```python
from build123d import *

# Parameters (mm, degrees)
SKETCH1_R                 = 5.5
BOSS_EXTRUDE1_DEPTH       = 6.35
F_6_CLEARANCE_HOLE1_D     = 3.7973
F_6_CLEARANCE_HOLE1_DEPTH = 6.35


with BuildPart() as part:
    # Sketch1 → Boss-Extrude1 (new body)
    with BuildSketch(Plane(origin=(0, 0, 0), x_dir=(0, 0, -1), z_dir=(1, 0, 0))):
        with BuildLine():
            Line((-19.05, 266.7), (19.05, 266.7))
            ThreePointArc((19.05, 266.7), (87.703033087, 128.539281009), (39.110598571, -17.88612161))
            ThreePointArc((39.110598571, -17.88612161), (37.900092771, -18.755241175), (36.426387255, -18.976341069))
            ThreePointArc((36.426387255, -18.976341069), (23.718766847, -12.493303526), (19.076049666, 0.995898429))
            ThreePointArc((19.076049666, 0.995898429), (19.289830149, 1.986417864), (19.804803607, 2.859133845))
            ThreePointArc((19.804803607, 2.859133845), (58.113146317, 140.316763388), (-19.05, 260.35))
            Line((-19.05, 260.35), (-19.05, 266.7))
        make_face()
        with Locations((38.1, 0)):
            Circle(SKETCH1_R, mode=Mode.SUBTRACT)
    extrude(amount=BOSS_EXTRUDE1_DEPTH)

    # #6 Clearance Hole1
    with Locations(Plane(origin=(6.35, 0, 0), x_dir=(0, 0, -1), z_dir=(1, 0, 0))):
        with Locations((-15.875, 263.525), (0, 263.525), (15.875, 263.525)):
            Hole(F_6_CLEARANCE_HOLE1_D / 2, depth=F_6_CLEARANCE_HOLE1_DEPTH)


solid = part.part
```
Geometry check sheet. Reference: the model listing, model coordinates, mm. Round coordinates to 2 decimals unless told otherwise and drop trailing zeros. Loops run counter-clockwise (first coordinate to the right, second up) from the corner with the lowest first, then second, coordinate; pieces in that order, holes last. Notation, with made-up numbers: (56.5, 69) - (74.5, 69) arc R32 cw to (74.5, 95) - close; hole circle Ø7 at (9, 37). An arc over 180 degrees is marked (long way). Use a Markdown table: item, result.
Q1. Cross-section at C-C on y = 194.5. Record the cut outline in (x, z).
Solutions:
| item | result |
|---|---|
| outline | (0, -71.65) - (6.35, -71.65) - (6.35, -40.53) - (0, -40.53) - close |
Q2. Material ranges on line 1 (Y direction, x = 1.5, z = -39); line 2 (Y direction, x = 4.25, z = -35); line 3 (Y direction, x = 4.5, z = 15), recorded low to high.
Solutions:
| item | result |
|---|---|
| line 1 | y = -18.01 to -5.43, 5.43 to 31.22, 197.38 to 246.61 |
| line 2 | y = -18.8 to -4.54, 4.54 to 24.23, 204.37 to 251.11 |
| line 3 | y = 257.63 to 261.84, 265.21 to 266.7 |
Q3. Draft check along Z on faces 1 (the cylindrical face through (3.131, -12.647, -23.854)), 2 (the flat face through (6.35, 125, -63)), 3 (the cylindrical face through (3.131, 130.749, -87.535)), 4 (the cylindrical face through (3.131, 0.242, -32.605)). Enter one of: released by +Z, released by -Z, zero draft, split by the parting line, or undercut.
Solutions:
| item | result |
|---|---|
| face 1 | released by +Z |
| face 2 | zero draft |
| face 3 | released by -Z |
| face 4 | undercut |
Q4. Cross-section at A-A on z = -24. Record the cut outline in (x, y), plus the area to 3 significant figures.
Solutions:
| item | result |
|---|---|
| outline | (0, -12.81) - (6.35, -12.81) - (6.35, 8.11) - (0, 8.11) - close; (0, 220.49) - (6.35, 220.49) - (6.35, 262.22) - (0, 262.22) - close |
| area | 398 mm2 |
Q5. Cross-section at D-D on z = -75. Record the cut outline in (x, y).
Solutions:
| item | result |
|---|---|
| outline | (0, 42.37) - (6.35, 42.37) - (6.35, 186.23) - (0, 186.23) - close |
Q6. Cross-section at B-B on x = 2. Record the cut outline in (y, z) (3 decimals), plus the area to 3 significant figures.
Solutions:
| item | result |
|---|---|
| outline | (-18.976, -36.426) arc R3.175 ccw to (-17.886, -39.111) arc R202.504 ccw to (266.7, -19.05) - (266.7, 19.05) - (260.35, 19.05) arc R174.365 cw to (2.859, -19.805) arc R3.175 ccw to (0.996, -19.076) arc R19.05 ccw to start; hole circle Ø11 at (0, -38.1); hole circle Ø3.797 at (263.525, -15.875); hole circle Ø3.797 at (263.525, 0); hole circle Ø3.797 at (263.525, 15.875) |
| area | 8,730 mm2 |
Q7. Go/stop test with flat-tipped pins: P1, Ø2, axis at x = 4.5, z = -14, coming from the -Y side; P2, Ø2.5, axis at y = 263.525, z = -15.875, coming from the +X side; P3, Ø2, axis at x = 3.5, y = 206, coming from the -Z side; P4, Ø2, axis at x = 4, z = 0.5, coming from the -Y side. Record where each tip stops, or that it passes through.
Solutions:
| item | result |
|---|---|
| P1 | stops at y = 231.28 |
| P2 | passes through |
| P3 | stops at z = -66.76 |
| P4 | stops at y = 245.54 |
